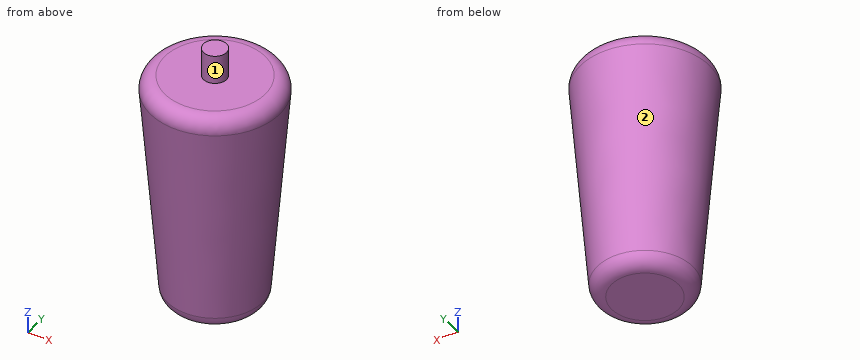
Autodesk Inventor part; units mm, degrees
ref_plane "作業平面2" through (0, 0, 81.7) normal (0, 0, 1) x (1, 0, 0)
ref_plane "YZ Plane" through (0, 0, 0) normal (1, 0, 0) x (0, 1, 0)
ref_plane "XZ Plane" through (0, 0, 0) normal (0, 1, 0) x (-1, 0, 0)
sketch "スケッチ1" plane through (0, 0, 0) normal (0, 0, 1) x (1, 0, 0)
  circle A0 centre (0, 0) radius 16.15
  dimension "d0" = 32.3
ref_plane "作業平面2" through (0, 0, 81.7) normal (0, 0, 1) x (1, 0, 0)
sketch "スケッチ3" plane through (0, 0, 81.7) normal (0, 0, 1) x (1, 0, 0)
  circle A0 centre (0, 0) radius 22.8
  dimension "d4" = 45.6
loft "ロフト1" add profiles "スケッチ3", "スケッチ1"
fillet "フィレット1" radius 5 2 edges at (-22.8, 0, 81.7) (-16.15, 0, 0)
sketch "スケッチ4" plane through (0, 0, 81.7) normal (0, 0, 1) x (1, 0, 0)
  circle A0 centre (0, 0) radius 4
  dimension "d10" = 8
extrude "押し出し1" add sketch "スケッチ4" along normal blind 10
properties part number "簡易ピーマン"
Verification items for the finished model (mm, model axes). Face numbers are marked on the shaded views. A direction names the side the tool comes from. Coordinates: 2 decimals unless noted, no trailing zeros. Write each loop counter-clockwise with the first axis right and the second up, starting at its lowest first coordinate (ties: lowest second). Pieces come first, ordered by that corner, then holes. Notation, with made-up numbers: M -37,68 L 7,68 A21 cw 7,95 Z; hole C 21,52.5 d7. An arc over 180 degrees is marked long. Answer as a JSON object with one key per item and string values. Group by question number.
(1) Cross-section at A-A, the plane x = 0. Record the cut outline in (y, z), and give its area (3 significant figures).
(2) Material ranges on line 1 (Y direction, x = 11.5, z = 49); line 2 (Z direction, x = 11.5, y = 1.5); line 3 (Z direction, x = -8, y = -14), recorded low to high.
(3) Gauge pin test, flat ends, axial feed: pin 1 (8 mm diameter, centred on x = -1.5, z = 47, fed in from +Y); pin 2 (1.5 mm diameter, centred on x = 17, z = 57, fed in from +Y); pin 3 (6 mm diameter, centred on x = -1, z = 46, fed in from -Y); pin 4 (2 mm diameter, centred on x = 18, y = 17.5, fed in from -Z). Record the tip position at first contact, or that the pin passes through.
(4) Cross-section at B-B, the plane z = 46. Record the cut outline in (x, y).
(5) Tool access check on the marked faces 1 and 2. Record the directions out of +Z, -Z, +X, -X, +Y, -Y that give a thin tool (end or side, any length) a straight path to the whole face; none if there is none.
Reply:
{
 "1": {"outline": "M -22.36,76.29 L -16.52,4.59 A5 ccw -11.54,0 L 11.54,0 A5 ccw 16.52,4.59 L 22.36,76.29 A5 ccw 17.38,81.7 L 4,81.7 L 4,91.7 L -4,91.7 L -4,81.7 L -17.38,81.7 A5 ccw Z", "area": "3,240 mm²"},
 "2": {"line 1": "-16.53 to 16.53", "line 2": "0 to 81.7", "line 3": "3 to 81.7"},
 "3": {"pin 1": "y = 20.28", "pin 2": "y = 12.97", "pin 3": "y = -20.13", "pin 4": "through"},
 "4": {"outline": "C 0,0 d39.79"},
 "5": {"face 1": "+Z", "face 2": "-Z"}
}
